from build123d import *

# Parameters (mm, degrees)
F1_DEPTH = 152.4
F2_W     = 133.35
F2_H     = 50.8
F3_DEPTH = 44.451
F4_R     = 6.35
F6_D     = 5.1054
F8_D     = 2.7051
F8_DEPTH = 15.08125
F8_TIP   = 0.8126940303


with BuildPart() as f1:
    # F0 (on Right) → F1 (new body)
    with BuildSketch(Plane.YZ):
        with BuildLine():
            ThreePointArc((-8.9046512, 76.2), (-23.9046512, 61.2), (-38.9046512, 76.2))
            Line((-38.9046512, 76.2), (-44.45, 76.2))
            Line((-44.45, 76.2), (-44.45, 0))
            Line((-44.45, 0), (-34.925, 0))
            Line((-34.925, 0), (-34.925, 1.4153871466))
            ThreePointArc((-34.925, 1.4153871466), (-39.6875, 12.7), (-34.925, 23.9846128534))
            Line((-34.925, 23.9846128534), (-34.925, 53.975))
            Line((-34.925, 53.975), (0, 53.975))
            Line((0, 53.975), (0, 76.2))
            Line((0, 76.2), (-8.9046512, 76.2))
        make_face()
    extrude(amount=F1_DEPTH)

    # F2 (on face) → F3 (cut, through all)
    with BuildSketch(Plane.XZ.offset(44.45)):
        with Locations((76.2, 50.8)):
            Rectangle(F2_W, F2_H)
    extrude(amount=-F3_DEPTH, mode=Mode.SUBTRACT)

    # F4
    f4_edges = [f1.edges().sort_by_distance(p)[0] for p in [
        (147.6375, 0, 53.975),
        (4.7625, 0, 53.975),
        (4.7625, -34.925, 53.975),
        (147.6375, -34.925, 53.975),
        (152.4, -39.6875, 0),
        (0, -39.6875, 0),
        (142.875, -39.6875, 25.4),
        (9.525, -39.6875, 25.4),
    ]]
    fillet(f4_edges, radius=F4_R)

    # F6 (through all)
    with Locations(Plane.XZ.offset(44.45)):
        with Locations((19.05, 12.7), (133.35, 12.7)):
            Hole(F6_D / 2)

    # F8
    with Locations(Plane.XY.offset(76.2)):
        with Locations((4.7625, -3.175), (4.7625, -41.275), (147.6375, -3.175), (147.6375, -41.4069328651)):
            Hole(F8_D / 2, depth=F8_DEPTH)
            with Locations((0, 0, -(F8_DEPTH + F8_TIP / 2))):  # 118° drill point
                Cone(0, F8_D / 2, F8_TIP, mode=Mode.SUBTRACT)


solid = f1.part
Part model, mm, in its own coordinate system. A direction names the side the tool comes from. Give positions to 0.01 mm unless a question says otherwise; leave off trailing zeros. Order: outer loops, then holes, each group sorted by start corner. A loop starts at its lowest first (then second) coordinate and runs counter-clockwise, first axis right, second up. Notation, with made-up numbers: (87, -33) - (125, -33) arc R19 cw to (125, 4) - close; hole circle Ø10 at (17.25, 59.25). An arc over 180 degrees is marked (long way). Use a Markdown table: item, result.
1) 3-axis set-ups, long thin cutter, end or side, ignore diameter. For faces 4 (the cylindrical face through (4.138, -42.475, 68.554)), 5 (the flat face through (5, -18, 53.975)), 6 (the cylindrical face through (11.336, -39.621, 27.31)): which of +Z, -Z, +X, -X, +Y, -Y reach the whole face in a straight line?
Checked values:
| item | result |
|---|---|
| face 4 | +Z |
| face 5 | -Z, +X, -X, +Y |
| face 6 | +Z, +Y, -Y |
2) Two-plate mould, pull along Y, no slides. Class faces 1 (the flat face through (148, -43, 76.2)), 2 (the flat face through (148, 0, 68)), 3 (the conical face through (4.979, -41.365, 60.447)): +Y half, -Y half, draft (parallel to the pull), parting line (faces both ways), or undercut.
Checked values:
| item | result |
|---|---|
| face 1 | draft |
| face 2 | +Y half |
| face 3 | undercut |
3) Flat gauge pins, fed straight in: P1, Ø1.6, axis at x = 94.5, z = 0.5, coming from the +Y side (3 decimals); P2, Ø2, axis at x = 147.64, y = -3.18, coming from the -Z side; P3, Ø7.5, axis at x = 5, y = -14, coming from the -Z side (3 decimals). Where does each tip first touch, or does it go through?
Checked values:
| item | result |
|---|---|
| P1 | y = -34.925 |
| P2 | z = 54.36 |
| P3 | z = 53.975 |
4) Saw through at D-D on y = -26. List the corners of the cut face in (x, z) (3 decimals).
Checked values:
| item | result |
|---|---|
| outline | (0, 53.975) - (9.525, 53.975) - (9.525, 61.347) - (0, 61.347) - close; (142.875, 53.975) - (152.4, 53.975) - (152.4, 61.347) - (142.875, 61.347) - close |
5) Saw through at A-A on z = 12.7. List the corners of the cut face in (x, y), plus the area to 3 significant figures.
Checked values:
| item | result |
|---|---|
| outline | (0, -44.45) - (16.5, -44.45) - (16.5, -39.69) - (0, -39.69) - close; (21.6, -44.45) - (130.8, -44.45) - (130.8, -39.69) - (21.6, -39.69) - close; (135.9, -44.45) - (152.4, -44.45) - (152.4, -39.69) - (135.9, -39.69) - close |
| area | 677 mm² |
6) Saw through at C-C on z = 69.5. Count the separate pieces of the cut face and the enclosed holes in it, plus the area to 3 significant figures.
Checked values:
| item | result |
|---|---|
| separate pieces | 4 |
| enclosed holes | 4 |
| area | 312 mm² |
7) Saw through at B-B on x = 19.05. List the corners of the cut face in (y, z) (3 decimals), plus the area to 3 significant figures.
Checked values:
| item | result |
|---|---|
| outline | (-44.45, 0) - (-34.925, 0) - (-34.925, 1.415) arc R15.751 cw to (-39.479, 10.147) - (-44.45, 10.147) - close; (-44.45, 15.253) - (-39.479, 15.253) arc R15.751 cw to (-34.925, 23.985) - (-34.925, 25.4) - (-44.45, 25.4) - close |
| area | 143 mm² |
8) Probe L1, parallel to X at y = -42.05, z = 12.7; L2, parallel to X at y = -41.5, z = 71.5 (3 decimals); L3, parallel to Z at x = 82, y = -43. List the from-to ranges inside material, lowest first. Write a range as from..to.
Checked values:
| item | result |
|---|---|
| L1 | 0..16.5, 21.6..130.8, 135.9..152.4 |
| L2 | 0..3.429, 6.096..9.525, 142.875..146.288, 148.987..152.4 |
| L3 | 0..25.4 |
